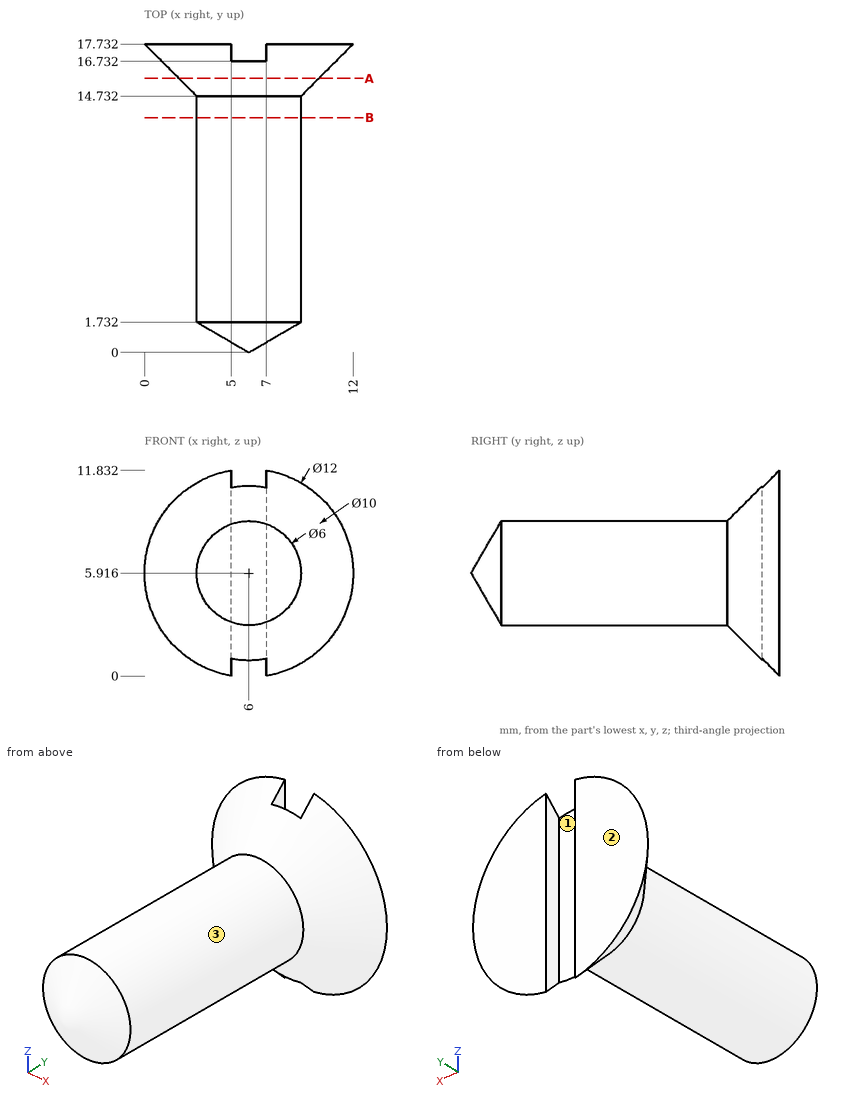
The drawing under review shows one solid part. Ordinate dimensions are in mm from its lowest x, y, z. A direction names the side the tool comes from. Coordinates: 2 decimals unless noted, no trailing zeros. Loops run counter-clockwise (first coordinate to the right, second up) from the corner with the lowest first, then second, coordinate; pieces in that order, holes last. Notation, with made-up numbers: (79.25, 55.5) - (125.25, 55.5) arc R21 cw to (125.25, 85.5) - close; hole circle Ø2 at (-8.75, 14). An arc over 180 degrees is marked (long way). Return JSON: item names as keys, results as strings.
Item 1: Take a section at B-B (y = 13.5). Give the boundary of the cut face in (x, z).
Determined:
{"outline": "circle Ø6 at (6, 5.92)"}
Item 2: For the marked faces 1, 2 and 3, list the 3-axis set-ups (+Z, -Z, +X, -X, +Y, -Y) from which the entire face can be reached by the end or side of a thin tool; tool diameter is ignored.
Determined:
{"face 1": "+Z, -Z, +Y", "face 2": "+Z, -Z, +X, -X, +Y", "face 3": "-Y"}
Item 3: Insertion check: pin 1 (0.6 mm diameter, centred on x = 6.5, z = 6, fed in from +Y); pin 2 (6 mm diameter, centred on x = 5.5, y = 7.5, fed in from -Z); pin 3 (5 mm diameter, centred on x = 2.5, y = 4, fed in from +Z). Each pin has a flat end and moves straight along its axis. Give the tip position at first contact, or say it passes through.
Determined:
{"pin 1": "stops at y = 16.73", "pin 2": "stops at z = 2.92", "pin 3": "stops at z = 8.74"}
Item 4: For line 1 (X direction, y = 17, z = 8.75); line 2 (Y direction, x = 6.25, z = 7.5); line 3 (Y direction, x = 4, z = 10.5), list the stretches that pass through material, from the lowest coordinate up.
Determined:
{"line 1": "x = 1.56 to 5, 7 to 10.44", "line 2": "y = 0.93 to 16.73", "line 3": "y = 16.73 to 17.73"}
Item 5: Take a section at A-A (y = 15.75). Give the boundary of the cut face in (x, z).
Determined:
{"outline": "circle Ø8.04 at (6, 5.92)"}
